Model file for the job. Use its own axes, mm. Face numbers are marked on the shaded views. A direction names the side the tool comes from. Round coordinates to 2 decimals unless told otherwise and drop trailing zeros. Order: outer loops, then holes, each group sorted by start corner. A loop starts at its lowest first (then second) coordinate and runs counter-clockwise, first axis right, second up. Notation, with made-up numbers: (66, 71) - (97, 71) arc R30 cw to (97, 110) - close; hole circle Ø6 at (-37.75, 68). An arc over 180 degrees is marked (long way). Answer as CSV lines item,"result". Start each with the question number.
1. Pull direction Y, two halves, no side cores. Call the marked faces 1, 2 and 3: released by +Y, released by -Y, zero draft, split by the parting line, or undercut.
2. Wall check: line 1 along Y through (x, z) = (-41, 7.5); line 2 along Z through (x, y) = (-23, 31); line 3 along X through (y, z) = (30, 1.25). Give the ranges that are in metal, low to high. Write a range as [from, to].
3. Pin check, flat tips, straight feed: pin 1 Ø4.5 at (y, z) = (28, 5) entering from -X; pin 2 Ø2 at (x, y) = (-56.5, 11.5) entering from +Z; pin 3 Ø2.5 at (x, z) = (-38, 6) entering from +Y; pin 4 Ø1.5 at (x, y) = (-27, 28.5) entering from -Z. Stop position of each tip, or through.
4. Band-saw the part on D-D on y = 34. List the corners of the cut face in (x, z).
5. Band-saw the part on A-A on z = 4.25. List the corners of the cut face in (x, y), then the cut area to 3 significant figures.
6. Band-saw the part on B-B on x = -37.5. List the corners of the cut face in (y, z).
7. 3-axis set-ups, long thin cutter, end or side, ignore diameter. For the marked faces 4, 5 and 6: which of +Z, -Z, +X, -X, +Y, -Y reach the whole face in a straight line?
8. Band-saw the part on C-C on y = 22. List the corners of the cut face in (x, z).
```python
from build123d import *

# Parameters (mm, degrees)
F0_R     = 0.5
F1_DEPTH = 8.7
F0_R_2   = 20
F2_DEPTH = 2.3
F3_DEPTH = 3


with BuildPart() as f1:
    # F0 (on Top) → F1 (new body)
    with BuildSketch(Plane.XY):
        with BuildLine():
            Line((-52.2276436281, 24.9724070162), (-52.2276436281, 28.9724070162))
            Line((-52.2276436281, 28.9724070162), (-54.2276436281, 28.9724070162))
            ThreePointArc((-54.2276436281, 28.9724070162), (-54.8130678601, 28.9293349241), (-55.3858843689, 28.8010462505))
            ThreePointArc((-55.3858843689, 28.8010462505), (-55.8776436281, 24.9724070162), (-55.3858843689, 21.1437677818))
            ThreePointArc((-55.3858843689, 21.1437677818), (-54.8130678601, 21.0154791082), (-54.2276436281, 20.9724070162))
            Line((-54.2276436281, 20.9724070162), (-52.2276436281, 20.9724070162))
            Line((-52.2276436281, 20.9724070162), (-52.2276436281, 24.9724070162))
        make_face()
        with Locations((-54.2276436281, 24.9724070162)):
            Circle(F0_R, mode=Mode.SUBTRACT)
        with Locations((-54.2276436281, 24.9724070162)):
            Circle(F0_R)
        with BuildLine():
            Line((-27.2276436281, 28.9724070162), (-29.2276436281, 28.9724070162))
            Line((-29.2276436281, 28.9724070162), (-29.2276436281, 24.9724070162))
            Line((-29.2276436281, 24.9724070162), (-29.2276436281, 20.9724070162))
            Line((-29.2276436281, 20.9724070162), (-27.2276436281, 20.9724070162))
            ThreePointArc((-27.2276436281, 20.9724070162), (-26.6422193961, 21.0154791082), (-26.0694028874, 21.1437677818))
            ThreePointArc((-26.0694028874, 21.1437677818), (-25.7010863507, 23.0423613201), (-25.5776436281, 24.9724070162))
            ThreePointArc((-25.5776436281, 24.9724070162), (-25.7010863507, 26.9024527122), (-26.0694028874, 28.8010462505))
            ThreePointArc((-26.0694028874, 28.8010462505), (-26.6422193961, 28.9293349241), (-27.2276436281, 28.9724070162))
        make_face()
        with BuildLine():
            ThreePointArc((-26.7276436281, 24.9724070162), (-27.2276436281, 24.4724070162), (-27.7276436281, 24.9724070162))
            ThreePointArc((-27.7276436281, 24.9724070162), (-27.2276436281, 25.4724070162), (-26.7276436281, 24.9724070162))
        make_face(mode=Mode.SUBTRACT)
        with BuildLine():
            ThreePointArc((-26.7276436281, 24.9724070162), (-27.2276436281, 25.4724070162), (-27.7276436281, 24.9724070162))
            ThreePointArc((-27.7276436281, 24.9724070162), (-27.2276436281, 24.4724070162), (-26.7276436281, 24.9724070162))
        make_face()
        with BuildLine():
            Line((-52.2276436281, 17.9224070162), (-52.2276436281, 20.9724070162))
            Line((-52.2276436281, 20.9724070162), (-54.2276436281, 20.9724070162))
            ThreePointArc((-54.2276436281, 20.9724070162), (-54.8130678601, 21.0154791082), (-55.3858843689, 21.1437677818))
            ThreePointArc((-55.3858843689, 21.1437677818), (-40.7276436281, 9.8224070162), (-26.0694028874, 21.1437677818))
            ThreePointArc((-26.0694028874, 21.1437677818), (-26.6422193961, 21.0154791082), (-27.2276436281, 20.9724070162))
            Line((-27.2276436281, 20.9724070162), (-29.2276436281, 20.9724070162))
            Line((-29.2276436281, 20.9724070162), (-29.2276436281, 17.9224070162))
            Line((-29.2276436281, 17.9224070162), (-52.2276436281, 17.9224070162))
        make_face()
        with BuildLine():
            Line((-52.2276436281, 28.9724070162), (-52.2276436281, 32.3224070162))
            Line((-52.2276436281, 32.3224070162), (-29.2276436281, 32.3224070162))
            Line((-29.2276436281, 32.3224070162), (-29.2276436281, 28.9724070162))
            Line((-29.2276436281, 28.9724070162), (-27.2276436281, 28.9724070162))
            ThreePointArc((-27.2276436281, 28.9724070162), (-26.6422193961, 28.9293349241), (-26.0694028874, 28.8010462505))
            ThreePointArc((-26.0694028874, 28.8010462505), (-40.7276436281, 40.1224070162), (-55.3858843689, 28.8010462505))
            ThreePointArc((-55.3858843689, 28.8010462505), (-54.8130678601, 28.9293349241), (-54.2276436281, 28.9724070162))
            Line((-54.2276436281, 28.9724070162), (-52.2276436281, 28.9724070162))
        make_face()
    extrude(amount=F1_DEPTH)

    # F0 (on Top) → F2 (join)
    with BuildSketch(Plane.XY):
        with Locations((-40.7276436281, 24.9724070162)):
            Circle(F0_R_2)
        with BuildLine():
            ThreePointArc((-55.3858843689, 21.1437677818), (-58.2276436281, 24.9724070162), (-55.3858843689, 28.8010462505))
            ThreePointArc((-55.3858843689, 28.8010462505), (-40.7276436281, 40.1224070162), (-26.0694028874, 28.8010462505))
            ThreePointArc((-26.0694028874, 28.8010462505), (-23.2276436281, 24.9724070162), (-26.0694028874, 21.1437677818))
            ThreePointArc((-26.0694028874, 21.1437677818), (-40.7276436281, 9.8224070162), (-55.3858843689, 21.1437677818))
        make_face(mode=Mode.SUBTRACT)
        with BuildLine():
            ThreePointArc((-55.3858843689, 21.1437677818), (-55.8776436281, 24.9724070162), (-55.3858843689, 28.8010462505))
            ThreePointArc((-55.3858843689, 28.8010462505), (-58.2276436281, 24.9724070162), (-55.3858843689, 21.1437677818))
        make_face()
        with BuildLine():
            ThreePointArc((-26.0694028874, 21.1437677818), (-23.2276436281, 24.9724070162), (-26.0694028874, 28.8010462505))
            ThreePointArc((-26.0694028874, 28.8010462505), (-25.7010863507, 26.9024527122), (-25.5776436281, 24.9724070162))
            ThreePointArc((-25.5776436281, 24.9724070162), (-25.7010863507, 23.0423613201), (-26.0694028874, 21.1437677818))
        make_face()
    extrude(amount=F2_DEPTH)

    # F0 (on Top) → F3 (cut)
    with BuildSketch(Plane.XY):
        with Locations((-54.2276436281, 24.9724070162)):
            Circle(F0_R)
        with BuildLine():
            ThreePointArc((-26.7276436281, 24.9724070162), (-27.2276436281, 25.4724070162), (-27.7276436281, 24.9724070162))
            ThreePointArc((-27.7276436281, 24.9724070162), (-27.2276436281, 24.4724070162), (-26.7276436281, 24.9724070162))
        make_face()
    extrude(amount=F3_DEPTH, mode=Mode.SUBTRACT)


solid = f1.part
```
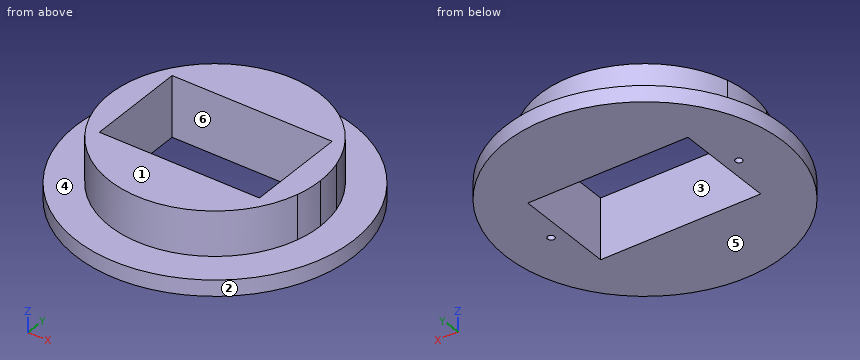
Reply:
1,face 1,"zero draft"
1,face 2,"split by the parting line"
1,face 3,"undercut"
2,line 1,"y = [9.82, 17.92], [32.32, 40.12]"
2,line 2,"z = [0, 2.3]"
2,line 3,"x = [-60.09, -52.23], [-29.23, -21.37]"
3,pin 1,"stops at x = -55.86"
3,pin 2,"stops at z = 2.3"
3,pin 3,"stops at y = 40.05"
3,pin 4,"stops at z = 0"
4,outline,"(-58.57, 0) - (-22.88, 0) - (-22.88, 2.3) - (-28.56, 2.3) - (-28.56, 8.7) - (-52.89, 8.7) - (-52.89, 2.3) - (-58.57, 2.3) - close"
5,outline,"circle Ø30.3 at (-40.73, 24.97); hole (-52.23, 17.92) - (-29.23, 17.92) - (-29.23, 32.32) - (-52.23, 32.32) - close"
5,area,"390 mm2"
6,outline,"(5.23, 0) - (17.92, 0) - (17.92, 8.7) - (10.17, 8.7) - (10.17, 2.3) - (5.23, 2.3) - close; (32.32, 0) - (44.71, 0) - (44.71, 2.3) - (39.77, 2.3) - (39.77, 8.7) - (32.32, 8.7) - close"
7,face 4,"+Z"
7,face 5,"-Z, +X, -X, +Y, -Y"
7,face 6,"+Z, -Z"
8,outline,"(-60.51, 0) - (-52.23, 0) - (-52.23, 8.7) - (-55.58, 8.7) - (-55.58, 2.3) - (-60.51, 2.3) - close; (-29.23, 0) - (-20.95, 0) - (-20.95, 2.3) - (-25.87, 2.3) - (-25.87, 8.7) - (-29.23, 8.7) - close"
